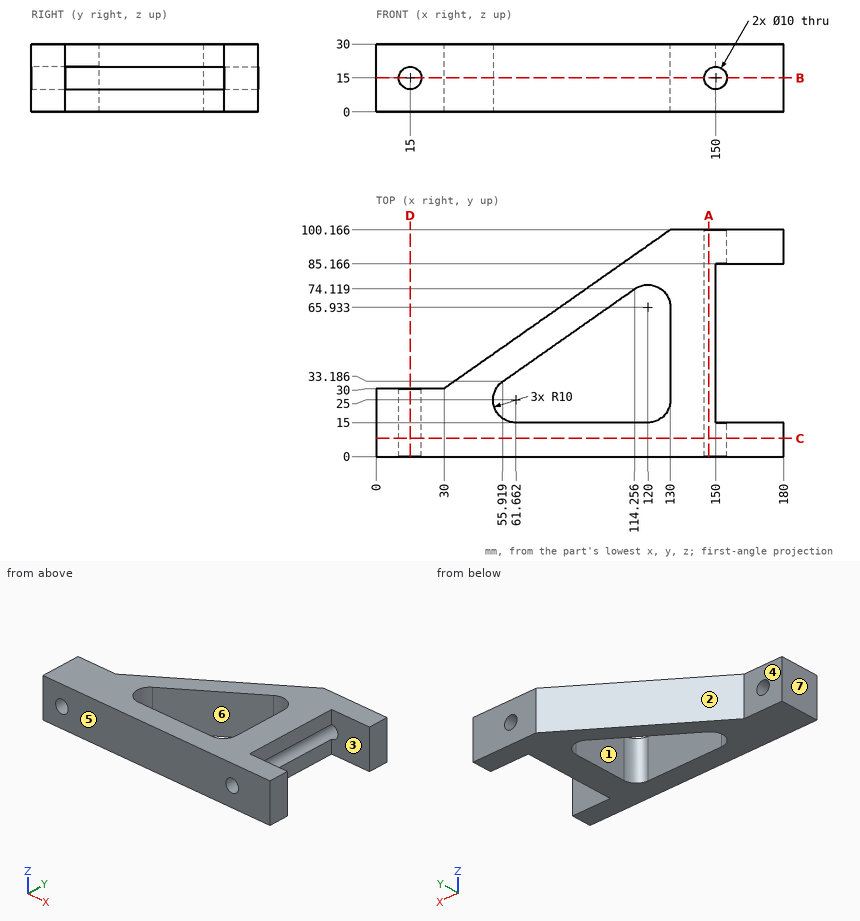
Input: dimensioned drawing with shaded views. Units: mm. Origin: part minimum x, y, z. A direction names the side the tool comes from. Round coordinates to 2 decimals unless told otherwise and drop trailing zeros. Loops run counter-clockwise (first coordinate to the right, second up) from the corner with the lowest first, then second, coordinate; pieces in that order, holes last.
1) Section query A-A on x = 147. Return the cut outline in (y, z) (1 decimal).
Ans:
outline: (0, 0) - (100.2, 0) - (100.2, 11) - (0, 11) - close; (0, 19) - (100.2, 19) - (100.2, 30) - (0, 30) - close
2) Section query B-B on z = 15. Return the cut outline in (x, y) (1 decimal).
Ans:
outline: (0, 0) - (10, 0) - (10, 30) - (0, 30) - close; (20, 0) - (145, 0) - (145, 100.2) - (130, 100.2) - (30, 30) - (20, 30) - close; (155, 0) - (180, 0) - (180, 15) - (155, 15) - close; (155, 85.2) - (180, 85.2) - (180, 100.2) - (155, 100.2) - close; hole (55.9, 33.2) arc R10 ccw to (61.7, 15) - (120, 15) arc R10 ccw to (130, 25) - (130, 65.9) arc R10 ccw to (114.3, 74.1) - close
3) Material intervals for line 1 (X direction, y = 14.75, z = 15); line 2 (X direction, y = 25, z = 15); line 3 (X direction, y = 25.5, z = 7.75) (1 decimal), sorted ascending.
Ans:
line 1: x = 0 to 10, 20 to 145, 155 to 180
line 2: x = 0 to 10, 20 to 51.66, 130 to 145
line 3: x = 0 to 51.7, 130 to 150
4) Pull-direction query (Y, two-part tool) for the marked faces 4, 5, 6 and 7; classes: released by +Y, released by -Y, zero draft, split by the parting line, or undercut.
Ans:
face 4: released by +Y
face 5: released by -Y
face 6: undercut
face 7: zero draft
5) Section query D-D on x = 15. Return the cut outline in (y, z), plus the area to 3 significant figures.
Ans:
outline: (0, 0) - (30, 0) - (30, 10) - (0, 10) - close; (0, 20) - (30, 20) - (30, 30) - (0, 30) - close
area: 600 mm2
6) Set-up query: the marked faces 1, 2 and 3. Return all of +Z, -Z, +X, -X, +Y, -Y with unobstructed straight access to the full face (end or side cutting, diameter ignored); none if empty.
Ans:
face 1: +Z, -Z
face 2: +Z, -Z, -X, +Y
face 3: +Z, -Z, +X
7) Pin query (flat end, axial travel): pin 1 (10 mm diameter, centred on y = 55.5, z = 23, fed in from +X); pin 2 (12 mm diameter, centred on y = 56.5, z = 7.5, fed in from -X) (1 decimal); pin 3 (15 mm diameter, centred on x = 84.5, z = 14.5, fed in from +Y); pin 4 (6 mm diameter, centred on x = 15, z = 15, fed in from -Y). Return the tip coordinate at first contact, or that it passes through.
Ans:
pin 1: stops at x = 150
pin 2: stops at x = 59.2
pin 3: stops at y = 73.5
pin 4: passes through
8) Section query C-C on y = 8. Return the cut outline in (x, z), plus the area to 3 significant figures.
Ans:
outline: (0, 0) - (180, 0) - (180, 30) - (0, 30) - close; hole circle Ø10 at (15, 15); hole circle Ø10 at (150, 15)
area: 5,240 mm2
